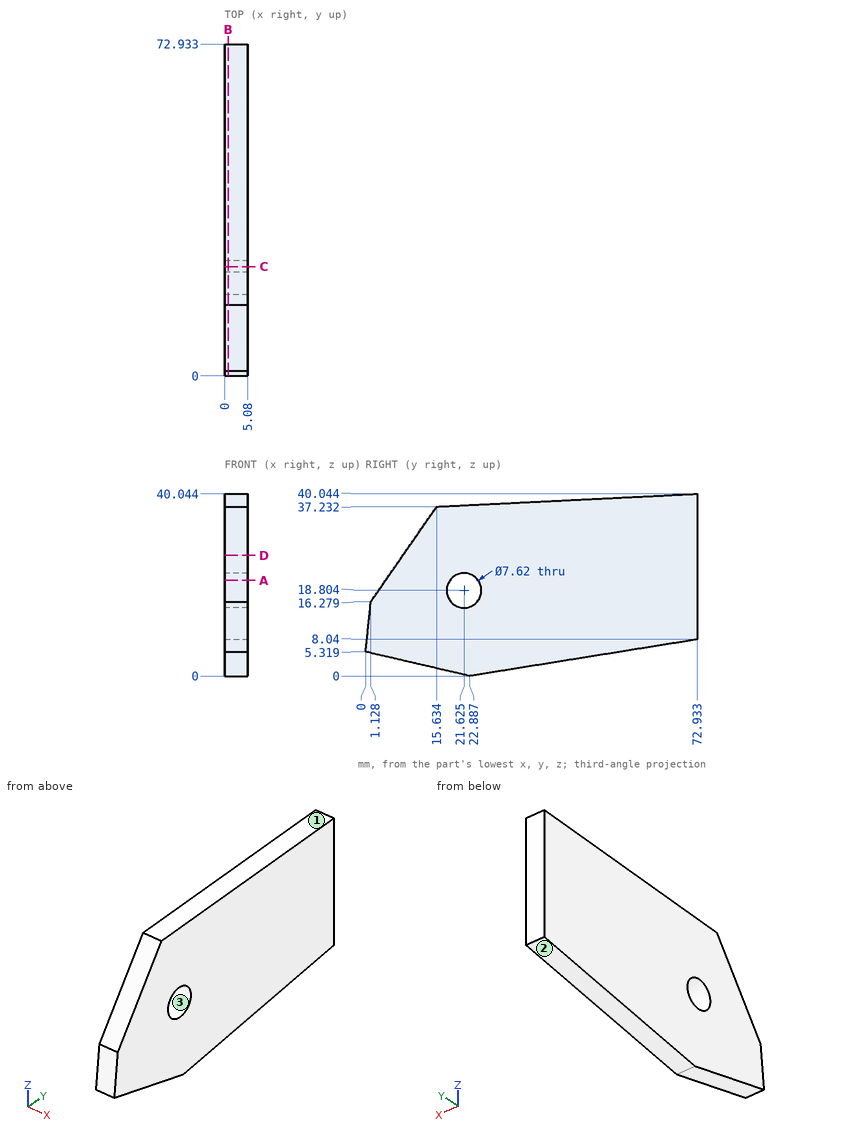
Could you check a few things on this drawing? It's one solid part, dimensions in mm from its lowest x, y, z. Round coordinates to 2 decimals unless told otherwise and drop trailing zeros. Order: outer loops, then holes, each group sorted by start corner. A loop starts at its lowest first (then second) coordinate and runs counter-clockwise, first axis right, second up.
(1) Imagine slicing it at C-C (y = 24). Write out the boundary of the cut face in (x, z) (1 decimal), plus the area to 3 significant figures.
Response values:
outline: (0, 0.2) - (5.1, 0.2) - (5.1, 15.8) - (0, 15.8) - close; (0, 21.8) - (5.1, 21.8) - (5.1, 37.6) - (0, 37.6) - close
area: 160 mm2
(2) If we mould it in two halves opening along Y, with no side actions, what happens to the marked faces 1, 2 and 3? For each: released by +Y, released by -Y, zero draft, split by the parting line, or undercut.
Response values:
face 1: released by -Y
face 2: released by +Y
face 3: undercut
(3) Imagine slicing it at A-A (z = 21). Write out the boundary of the cut face in (x, y).
Response values:
outline: (0, 4.4) - (5.08, 4.4) - (5.08, 18.51) - (0, 18.51) - close; (0, 24.74) - (5.08, 24.74) - (5.08, 72.93) - (0, 72.93) - close
(4) Imagine slicing it at B-B (x = 0.8). Write out the boundary of the cut face in (y, z) (1 decimal).
Response values:
outline: (0, 5.3) - (22.9, 0) - (72.9, 8) - (72.9, 40) - (15.6, 37.2) - (1.1, 16.3) - close; hole circle Ø7.6 at (21.6, 18.8)
(5) Imagine slicing it at D-D (z = 26.5). Write out the boundary of the cut face in (x, y) (1 decimal).
Response values:
outline: (0, 8.2) - (5.1, 8.2) - (5.1, 72.9) - (0, 72.9) - close
(6) I'm going to push flat-ended pins straight in: pin 1 (1.5 mm diameter, centred on x = 2, z = 24, fed in from -Y) (1 decimal); pin 2 (3 mm diameter, centred on x = 4.5, y = 41.5, fed in from -Z). Where does each tip first touch, or does it pass through?
Response values:
pin 1: stops at y = 6
pin 2: stops at z = 2.75
(7) Please list where these lines run through material, in increasing order: line 1 along Z through (x, y) = (4.8, 23.5); line 2 along Y through (x, z) = (2.1, 17); line 3 along Z through (x, y) = (0.8, 22) (1 decimal).
Response values:
line 1: z = 0.1 to 15.49, 22.12 to 37.62
line 2: y = 1.63 to 18.27, 24.98 to 72.93
line 3: z = 0.2 to 15, 22.6 to 37.5
